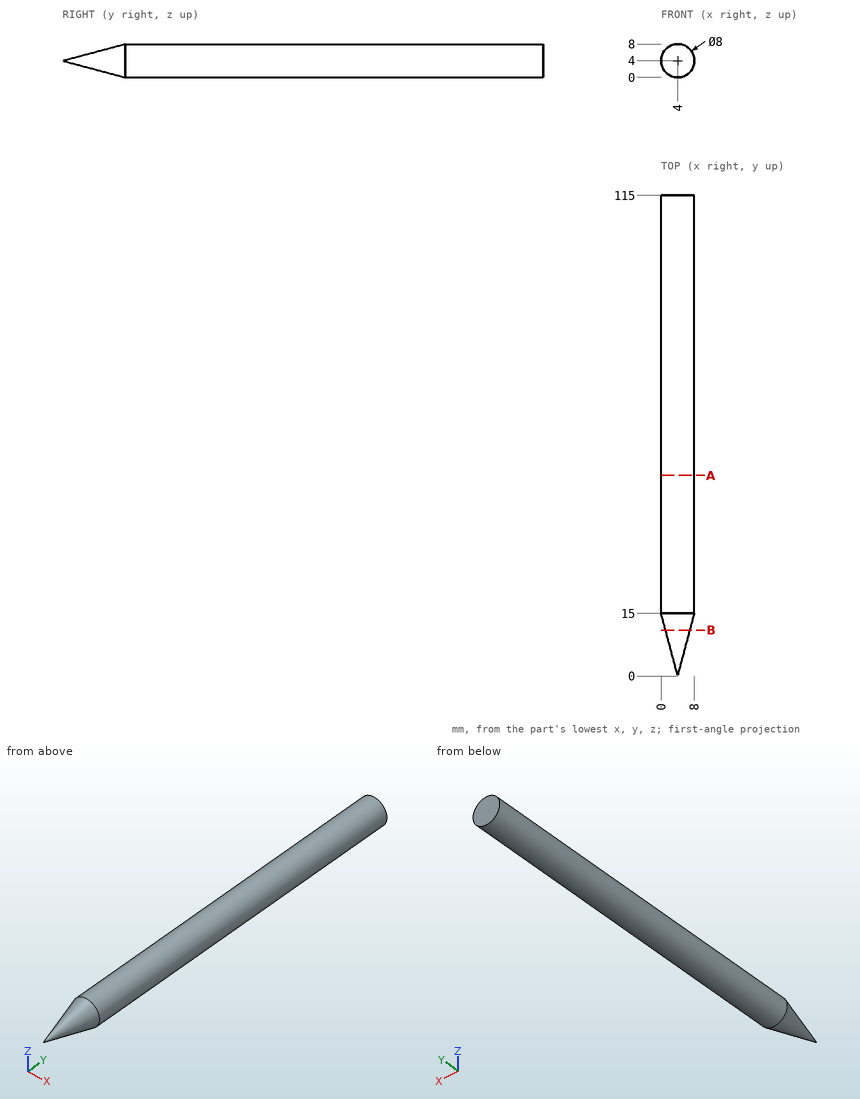
Job drawing, mm, ordinate dimensions from the low corner. One solid piece. Give positions to 0.01 mm unless a question says otherwise; leave off trailing zeros. Loops run counter-clockwise (first coordinate to the right, second up) from the corner with the lowest first, then second, coordinate; pieces in that order, holes last. Notation, with made-up numbers: (7, 62) -> (61, 62) arc R22 cw to (61, 76) -> close; hole circle Ø3 at (-29.5, -36). An arc over 180 degrees is marked (long way). Write each question's results on one line, items separated by ' | '. Start each with the question number.
Q1. Band-saw the part on A-A on y = 48. List the corners of the cut face in (x, z), plus the area to 3 significant figures.
Q2. Band-saw the part on B-B on y = 11. List the corners of the cut face in (x, z).
Q3. Pin check, flat tip, straight feed: P1, Ø1.5, axis at y = 65.5, z = 3, coming from the +X side. Stop position of the tip, or through.
Q4. Wall check: L1, parallel to X at y = 12.5, z = 2.75; L2, parallel to X at y = 23.5, z = 5.75; L3, parallel to Z at x = 7, y = 110. Give the ranges that are in metal, low to high.
Results are:
1) outline: circle Ø8 at (4, 4) | area: 50.3 mm²
2) outline: circle Ø5.87 at (4, 4)
3) P1: stops at x = 7.99
4) L1: x = 0.91 to 7.09 | L2: x = 0.4 to 7.6 | L3: z = 1.35 to 6.65
